Design review of the part built by this model. Coordinates are the model's own, in mm. Give positions to 0.01 mm unless a question says otherwise; leave off trailing zeros. Loops run counter-clockwise (first coordinate to the right, second up) from the corner with the lowest first, then second, coordinate; pieces in that order, holes last. Notation, with made-up numbers: M 67.25,83 L 126.25,83 A28 ccw 126.25,102 Z; hole C 37,62 d1. An arc over 180 degrees is marked long. Use one line per item in the form item = value. Start each with the question number.
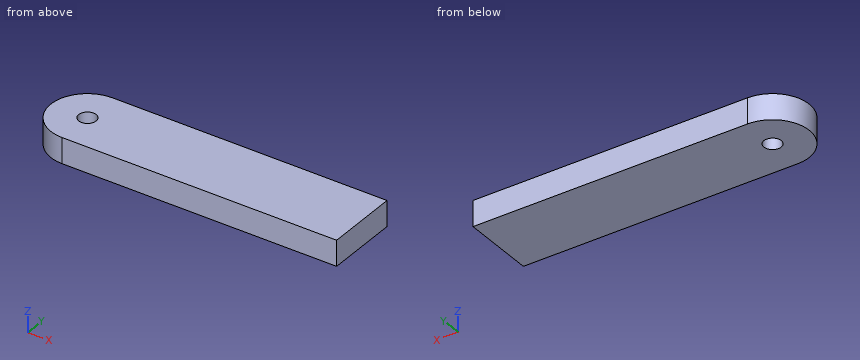
from build123d import *

# Parameters (mm, degrees)
SKETCH1_W               = 300
SKETCH1_H               = 80
BOSS_EXTRUDE1_DEPTH     = 28
SKETCH2_R               = 40
BOSS_EXTRUDE2_DEPTH     = 28
CUT_EXTRUDE2_DEPTH      = 312.743484294
CUT_EXTRUDE2_DEPTH_BACK = 312.743484294
SKETCH3_R               = 9.5


with BuildPart() as part:
    # Sketch1 → Boss-Extrude1 (new body)
    with BuildSketch(Plane.XY):
        with Locations((150, 40)):
            Rectangle(SKETCH1_W, SKETCH1_H)
    extrude(amount=BOSS_EXTRUDE1_DEPTH)

    # Sketch2 → Boss-Extrude2 (add)
    with BuildSketch(Plane.XY.offset(28)):
        with Locations((0, 40)):
            Circle(SKETCH2_R)
    extrude(amount=-BOSS_EXTRUDE2_DEPTH)

    # Sketch3 → Cut-Extrude2 (cut, two sides: drawn at the far end of the back side and taken through both)
    with BuildSketch(Plane.XY.offset(28).offset(-CUT_EXTRUDE2_DEPTH_BACK)):
        with Locations((0, 40)):
            Circle(SKETCH3_R)
    extrude(amount=CUT_EXTRUDE2_DEPTH + CUT_EXTRUDE2_DEPTH_BACK, mode=Mode.SUBTRACT)


solid = part.part
Q1. Wall thickness on probe 1 along X at (y, z) = (40, 13.75); probe 2 along Y at (x, z) = (0, 22); probe 3 along X at (y, z) = (41, 25): over which ranges is each line inside the solid? List them lowest first.
Q2. Take a section at C-C on y = 69. Give the boundary of the cut face in (x, z), plus the area to 3 significant figures.
Q3. Clearance check with flat-ended pins moving along their axes: pin 1 Ø4 at (x, y) = (233.5, 43.5) entering from -Z; pin 2 Ø4 at (y, z) = (38, 8) entering from -X; pin 3 Ø17 at (x, y) = (0, 40) entering from -Z; pin 4 Ø3 at (y, z) = (56.5, 13) entering from -X. State where each tip first meets the part, or that it passes through.
Q4. Take a section at B-B on z = 10.5. Give the boundary of the cut face in (x, y), plus the area to 3 significant figures.
Q5. Take a section at A-A on y = 40. Give the boundary of the cut face in (x, z), plus the area to 3 significant figures.
Response values:
q1.probe_1 = -40 to -9.5, 9.5 to 300
q1.probe_2 = 0 to 30.5, 49.5 to 80
q1.probe_3 = -39.99 to -9.45, 9.45 to 300
q2.outline = M -27.55,0 L 300,0 L 300,28 L -27.55,28 Z
q2.area = 9,170 mm^2
q3.pin_1 = 0
q3.pin_2 = -40
q3.pin_3 = through
q3.pin_4 = -37.08
q4.outline = M 0,0 L 300,0 L 300,80 L 0,80 A40 ccw Z; hole C 0,40 d19
q4.area = 26,200 mm^2
q5.outline = M -40,0 L -9.5,0 L -9.5,28 L -40,28 Z; M 9.5,0 L 300,0 L 300,28 L 9.5,28 Z
q5.area = 8,990 mm^2
